Can you work these out from the model? Positions are in its coordinate system, mm. A direction names the side the tool comes from. Round coordinates to 2 decimals unless told otherwise and drop trailing zeros. Order: outer loops, then holes, each group sorted by start corner. A loop starts at its lowest first (then second) coordinate and runs counter-clockwise, first axis right, second up. Notation, with made-up numbers: M 60.5,-23 L 112.5,-23 A14 ccw 112.5,4 Z; hole C 84.5,-33 d5. An arc over 180 degrees is marked long. Answer as CSV lines item,"result". Start each with the question number.
from build123d import *

# Parameters (mm, degrees)
BOSS_EXTRUDE1_DEPTH = 11.4808
SKETCH2_W           = 27.7114
SKETCH2_H           = 1.8034
CUT_EXTRUDE1_DEPTH  = 2.7432
SKETCH3_R           = 1.59385
CUT_EXTRUDE2_DEPTH  = 7.112
BOSS_EXTRUDE2_DEPTH = 11.4808
FILLET1_R           = 1.27
SKETCH5_W           = 7.2771
SKETCH5_H           = 0.64135
CUT_EXTRUDE3_DEPTH  = 1.27
CUT_EXTRUDE4_DEPTH  = 13.589


with BuildPart() as part:
    # Sketch1 → Boss-Extrude1 (new body)
    with BuildSketch(Plane.XY):
        Polygon((0, 0), (8.6741, 0), (8.6741, -1.2065), (13.5001, -1.2065), (13.5001, 0.8255), (20.7772, 0.8255), (20.7772, -1.2065), (27.7114, -1.2065), (27.7114, -11), (25.5016, -11), (25.5016, -9.0442), (15.7607, -9.0442), (15.7607, -11), (0, -11), align=None)
    extrude(amount=-BOSS_EXTRUDE1_DEPTH)

    # Sketch2 → Cut-Extrude1 (cut)
    with BuildSketch(Plane(origin=(0, 0.8255, 0), x_dir=(1, 0, 0), z_dir=(0, 1, 0))):
        with Locations((13.8557, 5.7404)):
            Rectangle(SKETCH2_W, SKETCH2_H)
    extrude(amount=-CUT_EXTRUDE1_DEPTH, mode=Mode.SUBTRACT)

    # Sketch3 → Cut-Extrude2 (cut)
    with BuildSketch(Plane(origin=(0, 0.8255, 0), x_dir=(1, 0, 0), z_dir=(0, 1, 0))):
        with Locations((17.13865, 9.06145)):
            Circle(SKETCH3_R)
        with Locations((17.13865, 2.41935)):
            Circle(SKETCH3_R)
    extrude(amount=-CUT_EXTRUDE2_DEPTH, mode=Mode.SUBTRACT)

    # Sketch4 → Boss-Extrude2 (add)
    with BuildSketch(Plane.XY):
        with BuildLine():
            Line((0, 10.844), (0, -11))
            Line((0, -11), (-17.78, -11))
            ThreePointArc((-17.78, -11), (-13.651034529, -0.078), (-17.78, 10.844))
            Line((-17.78, 10.844), (0, 10.844))
        make_face()
    extrude(amount=-BOSS_EXTRUDE2_DEPTH)

    # Fillet1
    fillet1_edges = [part.edges().sort_by_distance(p)[0] for p in [
        (-1.00965, -11, 0),
        (-1.00965, -11, -11.4808),
        (-8.89, 10.844, 0),
        (-13.651034529, -0.078, 0),
        (-13.651034529, -0.078, -11.4808),
        (-17.78, -11, -5.7404),
        (-8.89, 10.844, -11.4808),
        (-17.78, 10.844, -5.7404),
    ]]
    fillet(fillet1_edges, radius=FILLET1_R)

    # Sketch5 → Cut-Extrude3 (cut)
    with BuildSketch(Plane(origin=(0, 0.8255, 0), x_dir=(1, 0, 0), z_dir=(0, 1, 0))):
        with Locations((17.13865, 6.962775)):
            Rectangle(SKETCH5_W, SKETCH5_H)
        with Locations((17.13865, 11.160125)):
            Rectangle(SKETCH5_W, SKETCH5_H)
        with Locations((17.13865, 0.320675)):
            Rectangle(SKETCH5_W, SKETCH5_H)
        with Locations((17.13865, 4.518025)):
            Rectangle(SKETCH5_W, SKETCH5_H)
    extrude(amount=-CUT_EXTRUDE3_DEPTH, mode=Mode.SUBTRACT)

    # Sketch6 → Cut-Extrude4 (cut)
    with BuildSketch(Plane(origin=(27.7114, 0, 0), x_dir=(0, 0, -1), z_dir=(1, 0, 0))):
        with BuildLine():
            Line((3.1242, -11), (3.1242, -8.0282))
            ThreePointArc((3.1242, -8.0282), (5.7404, -5.412), (8.3566, -8.0282))
            Line((8.3566, -8.0282), (8.3566, -11))
            Line((8.3566, -11), (3.1242, -11))
        make_face()
    extrude(amount=-CUT_EXTRUDE4_DEPTH, mode=Mode.SUBTRACT)


solid = part.part
(1) For faces 4 (the flat face through (15, 0.826, -9)), 5 (the flat face through (21, -9.044, -2)), 6 (the flat face through (14.122, -8, -6)), which set-ups out of +Z, -Z, +X, -X, +Y, -Y let a thin tool reach every point of the face, with its end or its side?
(2) I want a section at A-A on x = 11.5. Write out the boundary of the cut face in (y, z), and give its area (3 significant figures).
(3) I'm going to push flat-ended pins straight in: P1, Ø1.6, axis at y = 0, z = -2.5, coming from the +X side; P2, Ø0.5, axis at x = 18.5, z = -4.5, coming from the +Y side; P3, Ø3.5, axis at x = 19, z = -1.5, coming from the -Y side. Where does each tip first touch, or does it pass through?
(4) I want a section at C-C on x = 22.5. Write out the boundary of the cut face in (y, z), and give its area (3 significant figures).
(5) If we mould it in two halves opening along X, with no side actions, what happens to faces 1 (the flat face through (-8, 10.844, -6)), 2 (the cylindrical face through (-13.65, -0.21, -5.68)), 3 (the flat face through (13.5, 0, -9))? For each: +X half, -X half, draft (parallel to the pull), parting line (faces both ways), or undercut.
(6) If I drill on line 1 along Z through (x, y) = (13, -1.75); line 2 along Y through (x, z) = (21, -1.5); line 3 along Y through (x, z) = (10.5, -4.75), over which ranges is the centre line in solid material (lowest first)?
(7) I want a section at B-B on z = -9.75. Write out the boundary of the cut face in (x, y).
(8) I want a section at D-D on y = -5. Count the separate pieces of the cut face and the enclosed holes in it, and give its area (3 significant figures).
From the geometry:
1,face 4,"+Z, -Z, +X, +Y"
1,face 5,"+Z, -Z, -Y"
1,face 6,"+X, -Y"
2,outline,"M -11,-10.21 A1.27 ccw -9.73,-11.48 L -1.21,-11.48 L -1.21,-6.64 L -1.92,-6.64 L -1.92,-4.84 L -1.21,-4.84 L -1.21,0 L -9.73,0 A1.27 ccw -11,-1.27 Z"
2,area,"110 mm²"
3,P1,"x = 20.78"
3,P2,"y = -0.44"
3,P3,"y = -9.04"
4,outline,"M -9.04,-11.48 L -1.21,-11.48 L -1.21,-6.64 L -1.92,-6.64 L -1.92,-4.84 L -1.21,-4.84 L -1.21,0 L -9.04,0 L -9.04,-3.12 L -8.03,-3.12 A2.62 cw -8.03,-8.36 L -9.04,-8.36 Z"
4,area,"72.6 mm²"
5,face 1,"draft"
5,face 2,"-X half"
5,face 3,"undercut"
6,line 1,"-11.48 to -6.64, -4.84 to 0"
6,line 2,"-9.04 to -1.21"
6,line 3,"-11 to -1.21"
7,outline,"M -16.3,-9.04 A1.27 ccw -15.23,-11 L 15.76,-11 L 15.76,-9.04 L 25.5,-9.04 L 25.5,-11 L 27.71,-11 L 27.71,-1.21 L 20.78,-1.21 L 20.78,0.83 L 18.58,0.83 L 18.58,-6.29 L 15.7,-6.29 L 15.7,0.83 L 13.5,0.83 L 13.5,-1.21 L 8.67,-1.21 L 8.67,0 L 0,0 L 0,10.84 L -15.23,10.84 A1.27 ccw -16.3,8.88 A16.51 cw Z"
8,separate pieces,"1"
8,enclosed holes,"2"
8,area,"467 mm²"
